from build123d import *

# Parameters (mm, degrees)
SKETCH1_R           = 30
SKETCH1_R_2         = 7
BOSS_EXTRUDE1_DEPTH = 10
FILLET1_R           = 10
FILLET2_R           = 20
CUT_EXTRUDE1_DEPTH  = 161.838428244


with BuildPart() as part:
    # Sketch1 → Boss-Extrude1 (new, symmetric)
    with BuildSketch(Plane(origin=(0, 0, 0), x_dir=(1, 0, 0), z_dir=(0, 1, 0))):
        with BuildLine():
            Line((27.935473676, 25.760615491), (128.063755469, 9.084385863))
            ThreePointArc((128.063755469, 9.084385863), (155, 0), (128.063755469, -9.084385863))
            Line((128.063755469, -9.084385863), (27.935473676, -25.760615491))
            ThreePointArc((27.935473676, -25.760615491), (-38, 0), (27.935473676, 25.760615491))
        make_face()
        with Locations(Location((0, 0, 0), (0, 0, 270))):
            Circle(SKETCH1_R, mode=Mode.SUBTRACT)
        with Locations(Location((140, 0, 0), (0, 0, 270))):
            Circle(SKETCH1_R_2, mode=Mode.SUBTRACT)
    extrude(amount=BOSS_EXTRUDE1_DEPTH, both=True)

    # Fillet1
    fillet1_edges = [part.edges().sort_by_distance(p)[0] for p in [
        (128.063755469, 0, -9.084385863),
        (128.063755469, 0, 9.084385863),
    ]]
    fillet(fillet1_edges, radius=FILLET1_R)

    # Fillet2
    fillet2_edges = [part.edges().sort_by_distance(p)[0] for p in [
        (27.935473676, 0, -25.760615491),
        (27.935473676, 0, 25.760615491),
    ]]
    fillet(fillet2_edges, radius=FILLET2_R)

    # Sketch2 → Cut-Extrude1 (cut, through all)
    with BuildSketch(Plane(origin=(0, 10, 0), x_dir=(1, 0, 0), z_dir=(0, 1, 0))):
        with BuildLine():
            Line((41.828554558, 17.870982725), (122.478416149, 4.438857582))
            ThreePointArc((122.478416149, 4.438857582), (126.238334256, -0.084646201), (122.310930345, -4.463523817))
            Line((122.310930345, -4.463523817), (41.652034204, -17.897153652))
            ThreePointArc((41.652034204, -17.897153652), (37.174066261, -16.149472145), (36.238855523, -11.43439331))
            ThreePointArc((36.238855523, -11.43439331), (38, 0), (36.238855523, 11.43439331))
            ThreePointArc((36.238855523, 11.43439331), (37.231968897, 16.217361812), (41.828554558, 17.870982725))
        make_face()
    extrude(amount=-CUT_EXTRUDE1_DEPTH, mode=Mode.SUBTRACT)


solid = part.part
Input: part model. Units: mm. Frame: model coordinates. A direction names the side the tool comes from. Coordinates: 2 decimals unless noted, no trailing zeros. Loops run counter-clockwise (first coordinate to the right, second up) from the corner with the lowest first, then second, coordinate; pieces in that order, holes last.
(1) Material intervals for probe 1 along X at (y, z) = (-3.25, 0); probe 2 along X at (y, z) = (0, -3.5); probe 3 along Z at (x, y) = (61.5, -2), sorted ascending.
(2) Section B-B on x = 0. Return the cut outline in (y, z), then the cut area to 3 significant figures.
(3) Section D-D on x = -23.5. Return the cut outline in (y, z), then the cut area to 3 significant figures.
(4) Section C-C on y = -2. Return the cut outline in (x, z), then the cut area to 3 significant figures.
(5) Section A-A on z = 0. Return the cut outline in (x, y), then the cut area to 3 significant figures.
(6) Set-up query: faces 1 (the face through (81.59, 0.14, -11.25)), 2 (the face through (37.5, 10, -3)), 3 (the face through (79.12, 0.14, 17.236)). Return all of +Z, -Z, +X, -X, +Y, -Y with unobstructed straight access to the full face (end or side cutting, diameter ignored); none if empty.
(7) Pull-direction query (Z, two-part tool) for faces 4 (the face through (1.32, -0.14, -29.97)), 5 (the face through (77.872, 0.14, -17.444)), 6 (the face through (28.79, 0.14, 26.35)); classes: released by +Z, released by -Z, zero draft, split by the parting line, or undercut.
(8) First-contact query: pin 1 Ø5 at (x, y) = (87, 5) entering from -Z; pin 2 Ø10 at (x, y) = (118.5, -4) entering from +Z; pin 3 Ø10 at (y, z) = (1, 8.5) entering from -X; pin 4 Ø11 at (x, z) = (140, 0) entering from +Y. Flat tips, straight axial feed; report the tip coordinate or a pass-through.
Data:
1. probe 1: x = -38 to -30, 30 to 38, 126.24 to 133, 147 to 155
1. probe 2: x = -37.84 to -29.8, 29.8 to 37.84, 124.57 to 133.94, 146.06 to 154.59
1. probe 3: z = -20.17 to -14.59, 14.59 to 20.17
2. outline: (-10, -38) - (10, -38) - (10, -30) - (-10, -30) - close; (-10, 30) - (10, 30) - (10, 38) - (-10, 38) - close
2. area: 320 mm2
3. outline: (-10, -29.86) - (10, -29.86) - (10, -18.65) - (-10, -18.65) - close; (-10, 18.65) - (10, 18.65) - (10, 29.86) - (-10, 29.86) - close
3. area: 449 mm2
4. outline: (24.38, -29.15) arc R20 cw to (33.92, -24.76) - (123.07, -9.92) arc R10 cw to (130.83, -11.87) arc R15 ccw (long way) to (130.83, 11.87) arc R10 cw to (123.07, 9.92) - (33.92, 24.76) arc R20 cw to (24.38, 29.15) arc R38 ccw (long way) to start; hole circle Ø60 at (0, 0); hole (36.24, -11.43) arc R5 ccw to (41.83, -17.87) - (122.48, -4.44) arc R4.5 ccw to (122.31, 4.46) - (41.65, 17.9) arc R5 ccw to (36.24, 11.43) arc R38 cw to start; hole circle Ø14 at (140, 0)
4. area: 3,380 mm2
5. outline: (-38, -10) - (-30, -10) - (-30, 10) - (-38, 10) - close; (30, -10) - (38, -10) - (38, 10) - (30, 10) - close; (126.24, -10) - (133, -10) - (133, 10) - (126.24, 10) - close; (147, -10) - (155, -10) - (155, 10) - (147, 10) - close
5. area: 615 mm2
6. face 1: +Y, -Y
6. face 2: +Z, -Z, +X, -X, +Y
6. face 3: +Z, +Y, -Y
7. face 4: undercut
7. face 5: released by -Z
7. face 6: released by +Z
8. pin 1: stops at z = -16.34
8. pin 2: stops at z = 11.51
8. pin 3: stops at x = -37.84
8. pin 4: passes through
